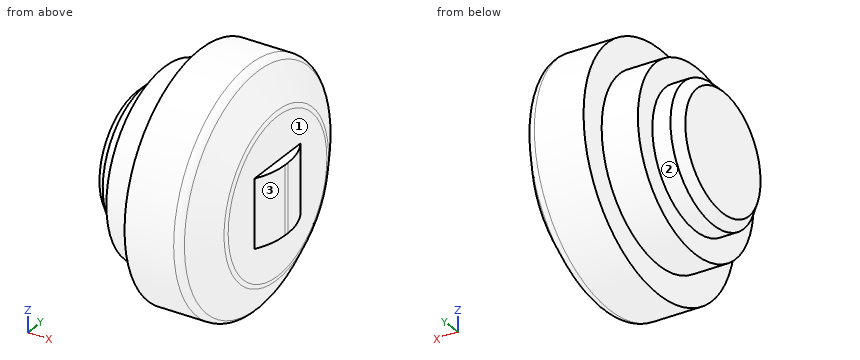
```python
from build123d import *

# Parameters (mm, degrees)
F3_SIZE     = 2
F4_SIZE2    = 8.6602540378
F4_SIZE     = 5
F5_R        = 2
F6_W        = 16
F6_H        = 15
F7_DEPTH    = 2
F8_T1_DEPTH = 52.4165738677


# Not quite as in the source:
# - a fillet or chamfer that OpenCascade refuses, or shapes differently, is made with other operations: its cross-section is extruded or revolved along the edge and cut away or added


with BuildPart() as f2:
    # F0 (on Front) → F2 (revolve)
    with BuildSketch(Plane.XZ):
        Polygon((0, 15), (0, 0), (31, 0), (31, 26.25), (14, 26.25), (14, 20), (6, 20), (6, 15), align=None)
    revolve(axis=Axis((43.7085926533, 0, 0), (1, 0, 0)))

    # F3
    f3_edges = [f2.edges().sort_by_distance(p)[0] for p in [
        (0, 0, -15),
    ]]
    chamfer(f3_edges, length=F3_SIZE)

    # F4
    f4_edges = [f2.edges().sort_by_distance(p)[0] for p in [
        (31, 0, -26.25),
    ]]
    chamfer(f4_edges, length=F4_SIZE, length2=F4_SIZE2)

    # F5
    f5_edges = [f2.edges().sort_by_distance(p)[0] for p in [
        (26, 0, -26.25),
        (31, 0, -17.589746),
    ]]
    fillet(f5_edges, radius=F5_R)

    # F6 (on face) → F7 (join)
    with BuildSketch(Plane.YZ.offset(31)):
        Rectangle(F6_W, F6_H)
    extrude(amount=F7_DEPTH)

    # F8: fillet of radius 15 on 2 edges, made by hand

    # F8_s2 → F8_t1 (cut)
    with BuildSketch(Plane.XY.offset(-26.2082869339)):
        with BuildLine():
            ThreePointArc((31, -8), (32.4913767462, -4.3896685727), (33, -0.5166852265))
            Line((33, -0.5166852265), (33, -8))
            Line((33, -8), (31, -8))
        make_face()
        with BuildLine():
            ThreePointArc((31, 8), (32.4913767462, 4.3896685727), (33, 0.5166852265))
            Line((33, 0.5166852265), (33, 8))
            Line((33, 8), (31, 8))
        make_face()
    extrude(amount=F8_T1_DEPTH, mode=Mode.SUBTRACT)


solid = f2.part
```
CAD build for the part. Positions are in the model's coordinates, mm. Face numbers are marked on the shaded views. A direction names the side the tool comes from. Round coordinates to 2 decimals unless told otherwise and drop trailing zeros. Write each loop counter-clockwise with the first axis right and the second up, starting at its lowest first coordinate (ties: lowest second). Pieces come first, ordered by that corner, then holes. Notation, with made-up numbers: (49, 30) -> (77, 30) arc R11 ccw to (77, 37) -> close; hole circle Ø1 at (0.25, 33.25). An arc over 180 degrees is marked (long way). Answer in a Markdown table with one row per item. Add a question column.
Item 1: Saw through at B-B, the plane x = 12.5. Write the cut outline in (y, z).
Item 2: Drill centre lines: line 1 (Z direction, x = 6.5, y = 0); line 2 (X direction, y = 14.5, z = 4); line 3 (X direction, y = 13.5, z = 2.5). Where is each one in solid material? Low to high. Write a range as from..to.
Item 3: Saw through at A-A, the plane x = 21.5. Write the cut outline in (y, z), then the cut area to 3 significant figures.
Item 4: Drop flat-ended pins along their axis: pin 1 Ø6 at (y, z) = (-8, 8.5) entering from -X; pin 2 Ø8 at (x, z) = (11, 7) entering from +Y; pin 3 Ø8 at (x, z) = (29.5, -8) entering from -Y; pin 4 Ø1.5 at (x, z) = (28.5, -4) entering from +Y. Give the stop position or say it passes through.
Item 5: Which spindle directions (+Z, -Z, +X, -X, +Y, -Y) get a long thin tool onto all of the face, cutting with end or side? Do the marked faces 1, 2 and 3. Say none if no direction does.
Findings below:
| question | item | result |
|---|---|---|
| 1 | outline | circle Ø40 at (0, 0) |
| 2 | line 1 | z = -20..20 |
| 2 | line 2 | x = 6..31 |
| 2 | line 3 | x = 0.73..31 |
| 3 | outline | circle Ø52.5 at (0, 0) |
| 3 | area | 2,160 mm^2 |
| 4 | pin 1 | stops at x = 0 |
| 4 | pin 2 | stops at y = 25.89 |
| 4 | pin 3 | stops at y = -25.19 |
| 4 | pin 4 | stops at y = 22.88 |
| 5 | face 1 | +X |
| 5 | face 2 | -X |
| 5 | face 3 | +Z, -Z, +X, -Y |
